```python
from build123d import *

# Parameters (mm, degrees)
SKETCH1_R           = 1.5875
BOSS_EXTRUDE1_DEPTH = 6.35
SKETCH3_R           = 1.5875
BOSS_EXTRUDE2_DEPTH = 6.35
FILLET1_R           = 3.175
BOSS_EXTRUDE3_START = -6.35
SKETCH4_R           = 3.175
SKETCH4_R_2         = 1.5875
BOSS_EXTRUDE3_DEPTH = 6.35
FILLET2_R           = 3.175
FILLET3_R           = 2.54


with BuildPart() as part:
    # Sketch1 → Boss-Extrude1 (new body)
    with BuildSketch(Plane.XY):
        with BuildLine():
            Line((13.97, -3.175), (39.37, -3.175))
            Line((39.37, -3.175), (56.515, -3.175))
            Line((56.515, -3.175), (56.515, 69.215))
            Line((56.515, 69.215), (41.625085175, 77.219758289))
            ThreePointArc((41.625085175, 77.219758289), (36.926481727, 77.112863097), (34.6075, 73.025))
            Line((34.6075, 73.025), (34.6075, 71.755))
            Line((34.6075, 71.755), (18.7325, 71.755))
            Line((18.7325, 71.755), (18.7325, 73.025))
            ThreePointArc((18.7325, 73.025), (16.413518273, 77.112863097), (11.714914825, 77.219758289))
            Line((11.714914825, 77.219758289), (-3.175, 69.215))
            Line((-3.175, 69.215), (-3.175, -3.175))
            Line((-3.175, -3.175), (13.97, -3.175))
        make_face()
        with Locations((35.56, 66.04)):
            Circle(SKETCH1_R, mode=Mode.SUBTRACT)
        with Locations((7.62, 66.04)):
            Circle(SKETCH1_R, mode=Mode.SUBTRACT)
        with Locations((50.8, 15.24)):
            Circle(SKETCH1_R, mode=Mode.SUBTRACT)
        with Locations((39.37, 73.025)):
            Circle(SKETCH1_R, mode=Mode.SUBTRACT)
        with Locations(Location((13.97, 73.025, 0), (0, 0, 180))):
            Circle(SKETCH1_R, mode=Mode.SUBTRACT)
        with BuildLine():
            Line((0, 11.093834149), (0, 16.5575))
            Line((0, 16.5575), (0, 66.04))
            Line((0, 66.04), (2.54, 66.04))
            Line((2.54, 66.04), (5.08, 63.506513025))
            ThreePointArc((5.08, 63.506513025), (8.990749111, 62.724701654), (11.2075, 66.04))
            Line((11.2075, 66.04), (11.2075, 68.58))
            Line((11.2075, 68.58), (31.9725, 68.58))
            Line((31.9725, 68.58), (31.9725, 66.04))
            ThreePointArc((31.9725, 66.04), (35.56, 62.4525), (39.1475, 66.04))
            Line((39.1475, 66.04), (40.386, 66.04))
            Line((40.386, 66.04), (53.34, 66.04))
            Line((53.34, 66.04), (53.34, 18.415))
            Line((53.34, 18.415), (50.8, 18.415))
            ThreePointArc((50.8, 18.415), (47.625, 15.24), (50.8, 12.065))
            Line((50.8, 12.065), (53.34, 12.065))
            Line((53.34, 12.065), (53.34, 0))
            Line((53.34, 0), (0, 0))
            Line((0, 0), (0, 11.093834149))
        make_face(mode=Mode.SUBTRACT)
    extrude(amount=BOSS_EXTRUDE1_DEPTH)

    # Sketch3 → Boss-Extrude2 (add)
    # profile 1 of 2: a face of its own
    with BuildSketch(Plane.XY.offset(6.35)):
        with BuildLine():
            Line((-7.423658, 10.969244), (-3.175, 10.969244))
            Line((-3.175, 10.969244), (-3.175, 3.031744))
            Line((-3.175, 3.031744), (-7.423658, 3.031744))
            ThreePointArc((-7.423658, 3.031744), (-11.392408, 7.000494), (-7.423658, 10.969244))
        make_face()
        with Locations((-7.423658, 7.000494)):
            Circle(SKETCH3_R, mode=Mode.SUBTRACT)
    # profile 2 of 2: a face of its own
    with BuildSketch(Plane.XY.offset(6.35)):
        with BuildLine():
            Line((56.515, 3.031744), (56.515, 10.969244))
            Line((56.515, 10.969244), (60.763658, 10.969244))
            ThreePointArc((60.763658, 10.969244), (64.732408, 7.000494), (60.763658, 3.031744))
            Line((60.763658, 3.031744), (56.515, 3.031744))
        make_face()
        with Locations((60.763658, 7.000494)):
            Circle(SKETCH3_R, mode=Mode.SUBTRACT)
    extrude(amount=-BOSS_EXTRUDE2_DEPTH)

    # Fillet1
    fillet1_edges = [part.edges().sort_by_distance(p)[0] for p in [
        (56.515, 3.031744, 3.175),
        (56.515, 10.969244, 3.175),
        (-3.175, 10.969244, 3.175),
        (-3.175, 3.031744, 3.175),
    ]]
    fillet(fillet1_edges, radius=FILLET1_R)

    # Sketch4 → Boss-Extrude3 (add)
    # profile 1 of 4: a face of its own
    with BuildSketch(Plane.XY.offset(6.35).offset(BOSS_EXTRUDE3_START)):
        with BuildLine():
            Line((-4.164100811, 77.557794463), (-3.175, 69.215))
            Line((-3.175, 69.215), (11.714914825, 77.219758289))
            ThreePointArc((11.714914825, 77.219758289), (12.807272625, 77.643384057), (13.97, 77.7875))
            Line((13.97, 77.7875), (6.640337345, 80.156211745))
            ThreePointArc((6.640337345, 80.156211745), (0.583964497, 84.374611001), (-4.318131733, 78.857003104))
            Line((-4.318131733, 78.857003104), (-4.164100811, 77.557794463))
        make_face()
        with Locations((1.238118267, 78.857003104)):
            Circle(SKETCH4_R, mode=Mode.SUBTRACT)
    # profile 2 of 4: a face of its own
    with BuildSketch(Plane.XY.offset(6.35).offset(BOSS_EXTRUDE3_START)):
        with BuildLine():
            Line((41.625085175, 77.219758289), (56.515, 69.215))
            Line((56.515, 69.215), (57.504100811, 77.557794463))
            Line((57.504100811, 77.557794463), (57.658131733, 78.857003104))
            ThreePointArc((57.658131733, 78.857003104), (52.756035503, 84.374611001), (46.699662655, 80.156211745))
            Line((46.699662655, 80.156211745), (39.37, 77.7875))
            ThreePointArc((39.37, 77.7875), (40.532727375, 77.643384057), (41.625085175, 77.219758289))
        make_face()
        with Locations((52.101881733, 78.857003104)):
            Circle(SKETCH4_R, mode=Mode.SUBTRACT)
    # profile 3 of 4: a face of its own
    with BuildSketch(Plane.XY.offset(6.35).offset(BOSS_EXTRUDE3_START)):
        with BuildLine():
            Line((56.515, 47.137146639), (56.515, 39.199646639))
            Line((56.515, 39.199646639), (59.69, 39.199646639))
            ThreePointArc((59.69, 39.199646639), (63.65875, 43.168396639), (59.69, 47.137146639))
            Line((59.69, 47.137146639), (56.515, 47.137146639))
        make_face()
        with Locations((59.69, 43.168396639)):
            Circle(SKETCH4_R_2, mode=Mode.SUBTRACT)
    # profile 4 of 4: a face of its own
    with BuildSketch(Plane.XY.offset(6.35).offset(BOSS_EXTRUDE3_START)):
        with BuildLine():
            Line((-3.175, 47.137146639), (-6.35, 47.137146639))
            ThreePointArc((-6.35, 47.137146639), (-10.31875, 43.168396639), (-6.35, 39.199646639))
            Line((-6.35, 39.199646639), (-3.175, 39.199646639))
            Line((-3.175, 39.199646639), (-3.175, 47.137146639))
        make_face()
        with Locations((-6.35, 43.168396639)):
            Circle(SKETCH4_R_2, mode=Mode.SUBTRACT)
    extrude(amount=BOSS_EXTRUDE3_DEPTH)

    # Fillet2
    fillet2_edges = [part.edges().sort_by_distance(p)[0] for p in [
        (46.699662655, 80.156211745, 3.175),
        (6.640337345, 80.156211745, 3.175),
        (-3.175, 47.137146639, 3.175),
        (56.515, 47.137146639, 3.175),
        (56.515, 39.199646639, 3.175),
        (-3.175, 39.199646639, 3.175),
    ]]
    fillet(fillet2_edges, radius=FILLET2_R - 0.0001)  # a hair under: the kernel refuses the full size

    # Fillet3
    fillet3_edges = [part.edges().sort_by_distance(p)[0] for p in [
        (-3.175, 69.215, 3.175),
        (13.97, 77.7875, 3.175),
        (56.515, 69.215, 3.175),
        (39.37, 77.7875, 3.175),
    ]]
    fillet(fillet3_edges, radius=FILLET3_R)


solid = part.part
```
Input: part model. Units: mm. Frame: model coordinates. A direction names the side the tool comes from. Round coordinates to 2 decimals unless told otherwise and drop trailing zeros. Loops run counter-clockwise (first coordinate to the right, second up) from the corner with the lowest first, then second, coordinate; pieces in that order, holes last. Notation, with made-up numbers: (-23.5, -20) - (18.5, -20) arc R21 cw to (18.5, 17) - close; hole circle Ø2 at (-33.75, 24). An arc over 180 degrees is marked (long way). One line per item, written item: value. Start each with the question number.
(1) Section A-A, the plane y = 15.24. Count the separate pieces of the cut face and the enclosed holes in it, plus the area to 3 significant figures.
(2) Draft query along Y for faces 1 (the cylindrical face through (46.329, 80.294, 3.219)), 2 (the cylindrical face through (60.42, 41.76, 3.13)). Return one class per face: +Y half, -Y half, draft (parallel to the pull), parting line (faces both ways), or undercut.
(3) Section D-D, the plane x = 17.5. Return loops of the section in (y, z) (3 decimals), plus the area to 3 significant figures.
(4) Section C-C, the plane y = 54.5. Return loops of the section in (x, z) (3 decimals).
(5) Access query for faces 3 (the flat face through (52, 18.415, 3)), 4 (the flat face through (56.515, 60, 3)), 5 (the cylindrical face through (-4.08, 11.924, 3.131)). Directions: +Z, -Z, +X, -X, +Y, -Y. A direction counts if a zero-diameter tool reaches every point of the face in a straight line with its end or side. Return the directions, or none.
(6) Contact query for flat-ended pins moving along their axis: P1, Ø0.9, axis at x = -6.5, z = 4, coming from the +Y side; P2, Ø1, axis at x = -2.5, z = 2.5, coming from the +Y side; P3, Ø3, axis at x = 39.37, y = 73.025, coming from the -Z side; P4, Ø8, axis at x = -1.5, y = 66, coming from the -Z side. Output: stop coordinate, or through.
(7) Ray query, line 1 (X direction, y = 53.5, z = 4.75) (3 decimals); line 2 (X direction, y = 44, z = 4); line 3 (X direction, y = 80.5, z = 3.5). Return the intervals inside material, ascending. Write a range as [from, to].
Results below:
1. separate pieces: 3
1. enclosed holes: 0
1. area: 56.5 mm^2
2. face 1: +Y half
2. face 2: undercut
3. outline: (-3.175, 0) - (0, 0) - (0, 6.35) - (-3.175, 6.35) - close; (68.58, 0) - (76.222, 0) - (76.222, 6.35) - (68.58, 6.35) - close
3. area: 68.7 mm^2
4. outline: (-3.175, 0) - (0, 0) - (0, 6.35) - (-3.175, 6.35) - close; (53.34, 0) - (56.515, 0) - (56.515, 6.35) - (53.34, 6.35) - close
5. face 3: +Z, -Z
5. face 4: +Z, -Z, +X
5. face 5: +Z, -Z, -X
6. P1: y = 47.15
6. P2: y = 83.37
6. P3: through
6. P4: z = 0
7. line 1: [-3.175, 0], [53.34, 56.515]
7. line 2: [-10.23, -7.7], [-5, 0], [53.34, 58.34], [61.04, 63.57]
7. line 3: [-4.07, -1.48], [3.95, 6.79], [46.55, 49.39], [54.82, 57.41]
